The drawing under review shows one solid part. Ordinate dimensions are in mm from its lowest x, y, z. Coordinates: 2 decimals unless noted, no trailing zeros. Write each loop counter-clockwise with the first axis right and the second up, starting at its lowest first coordinate (ties: lowest second). Pieces come first, ordered by that corner, then holes.
1) Mouldability with a two-part tool opening along Y and no side actions: class the marked faces 1 and 2 as pulls with the +Y half, pulls with the -Y half, needs draft (parallel to the pull), parting line crosses it, or undercut.
2) To check wall thickness, follow line 1 along Z through (x, y) = (63.5, 2.05); line 2 along X through (y, z) = (4.1, 8); line 3 along X through (y, z) = (4.55, 92) (1 decimal). State the ranges of each line that lie inside material, in increasing order.
3) We need section C-C on z = 49. Write out the cut boundary in (x, y), then the cut area to 3 significant figures.
4) We need section B-B on y = 3.6. Write out the cut boundary in (x, z).
5) We need section D-D on x = 34. Write out the cut boundary in (y, z).
6) Insertion check: P1, Ø1.5, axis at x = 77, y = 3, coming from the +Z side; P2, Ø1, axis at y = 4.5, z = 65, coming from the +X side; P3, Ø1.5, axis at x = 24.5, y = 3.5, coming from the -Z side; P4, Ø7, axis at x = 34, z = 89.3, coming from the -Y side. Each pin has a flat end and moves straight along its axis. Give the tip position at first contact, or say it passes through.
7) We need section A-A on x = 49. Write out the cut boundary in (y, z).
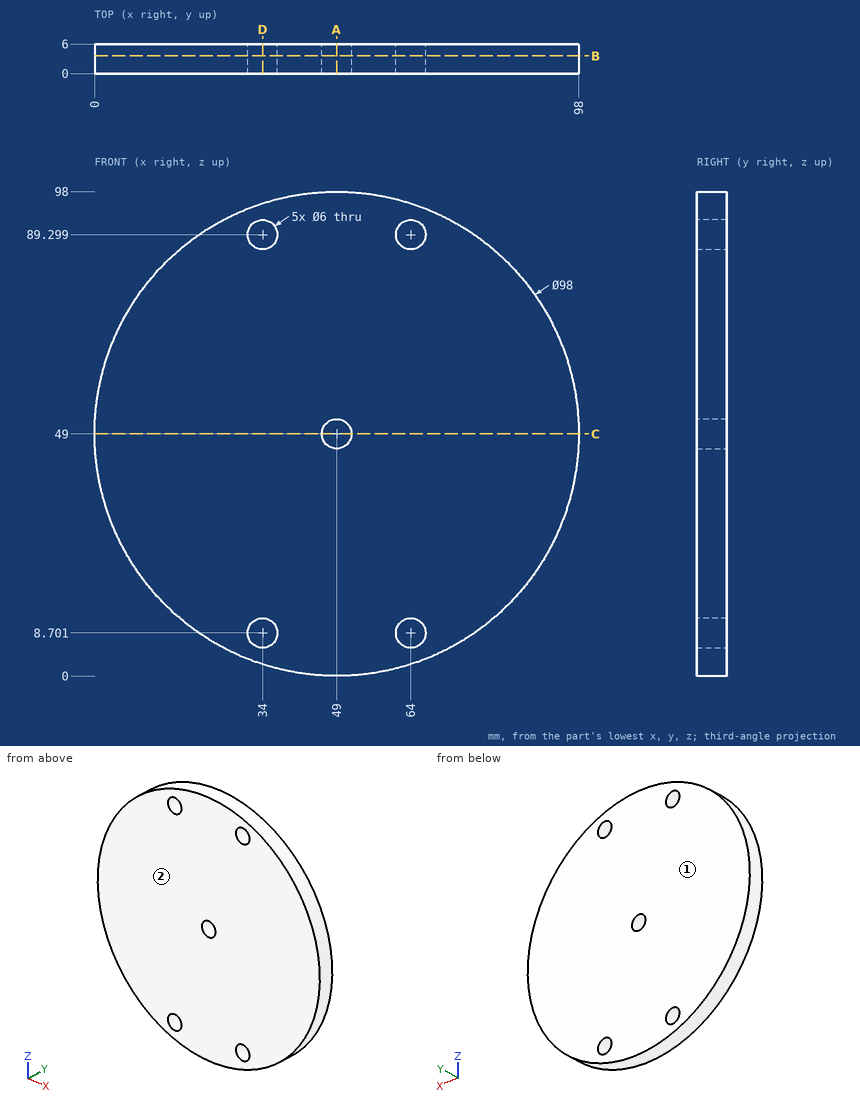
Result:
1. face 1: pulls with the +Y half
1. face 2: pulls with the -Y half
2. line 1: z = 2.19 to 5.74, 11.66 to 86.34, 92.26 to 95.81
2. line 2: x = 22.17 to 31.08, 36.92 to 61.08, 66.92 to 75.83
2. line 3: x = 25.5 to 32.7, 35.3 to 62.7, 65.3 to 72.5
3. outline: (0, 0) - (46, 0) - (46, 6) - (0, 6) - close; (52, 0) - (98, 0) - (98, 6) - (52, 6) - close
3. area: 552 mm2
4. outline: circle Ø98 at (49, 49); hole circle Ø6 at (34, 8.7); hole circle Ø6 at (34, 89.3); hole circle Ø6 at (49, 49); hole circle Ø6 at (64, 8.7); hole circle Ø6 at (64, 89.3)
5. outline: (0, 2.35) - (6, 2.35) - (6, 5.7) - (0, 5.7) - close; (0, 11.7) - (6, 11.7) - (6, 86.3) - (0, 86.3) - close; (0, 92.3) - (6, 92.3) - (6, 95.65) - (0, 95.65) - close
6. P1: stops at z = 89.72
6. P2: stops at x = 95.48
6. P3: stops at z = 6.14
6. P4: stops at y = 0
7. outline: (0, 0) - (6, 0) - (6, 46) - (0, 46) - close; (0, 52) - (6, 52) - (6, 98) - (0, 98) - close
